Answer from the drawing. Dimensions are ordinates in mm from the lowest x, y and z of the part. A direction names the side the tool comes from. Coordinates: 2 decimals unless noted, no trailing zeros. Write each loop counter-clockwise with the first axis right and the second up, starting at its lowest first coordinate (ties: lowest second). Pieces come first, ordered by that corner, then holes.
(1) The part is cut by section B-B, the plane z = 1.5. State how many separate pieces and enclosed holes the cut face has, and give its area (3 significant figures).
(2) Given pin 1 (1.5 mm diameter, centred on x = 15.5, z = 4, fed in from -Y); pin 2 (3 mm diameter, centred on x = 13, z = 2, fed in from +Y); pin 3 (3 mm diameter, centred on x = 2, z = 2.5, fed in from +Y), each flat-ended and moving along its own axis, determine where each tip first touches the part or whether it passes through.
(3) The part is cut by section C-C, the plane x = 13.5. Determine the outline of the cut face in (y, z).
(4) The part is cut by section D-D, the plane x = 34. Determine the outline of the cut face in (y, z).
(5) Straight lines are drawn through the part: line 1 along X through (y, z) = (58.5, 4); line 2 along X through (y, z) = (39.5, 2.5) (1 decimal); line 3 along Y through (x, z) = (29.5, 5.5) (1 decimal). For each, find the intervals that lie inside material, in ascending order.
(6) The part is cut by section A-A, the plane x = 3. Determine the outline of the cut face in (y, z), and give its area (3 significant figures).
(7) Determine the mould class of the marked faces 1, 2 and 3 for opening direction Y: pulls with the +Y half, pulls with the -Y half, needs draft (parallel to the pull), parting line crosses it, or undercut.
(8) Which of the six approach directions +Z, -Z, +X, -X, +Y, -Y give full straight-line access (tool end or side, diameter ignored) to the marked faces 4 and 5?
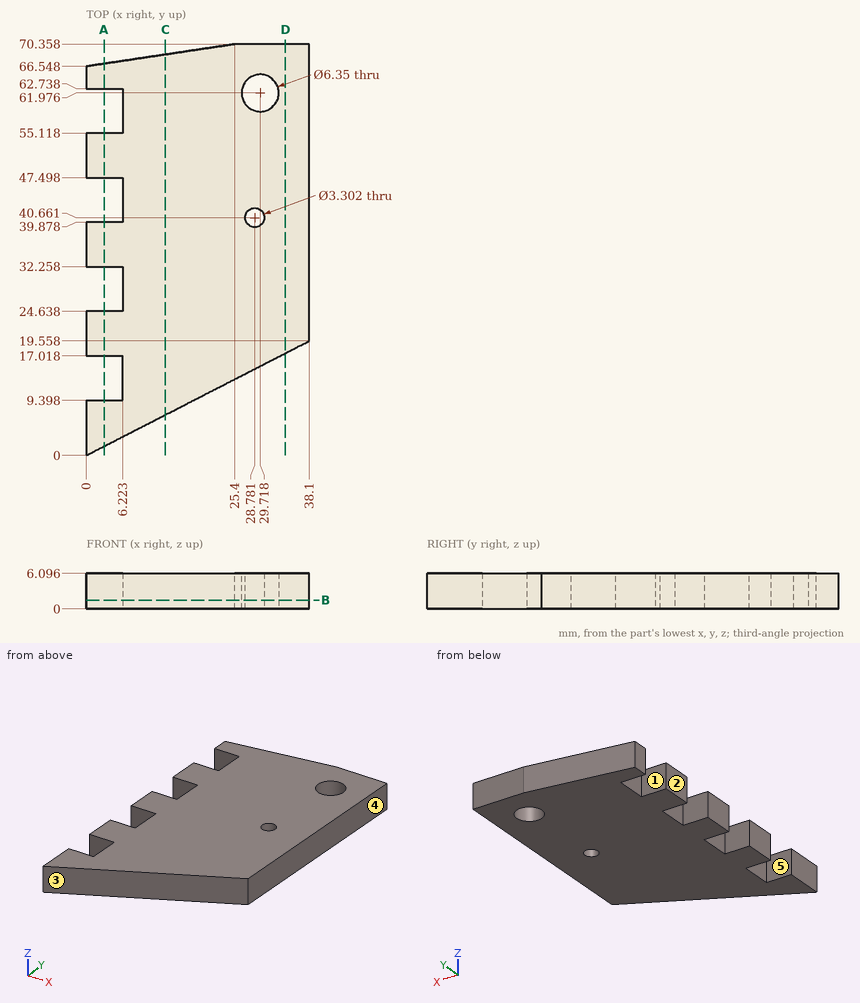
Computed:
1. separate pieces: 1
1. enclosed holes: 2
1. area: 2,030 mm2
2. pin 1: stops at y = 7.57
2. pin 2: stops at y = 68.72
2. pin 3: stops at y = 67.07
3. outline: (6.93, 0) - (68.57, 0) - (68.57, 6.1) - (6.93, 6.1) - close
4. outline: (17.45, 0) - (70.36, 0) - (70.36, 6.1) - (17.45, 6.1) - close
5. line 1: x = 6.22 to 38.1
5. line 2: x = 0 to 27.6, 30 to 38.1
5. line 3: y = 15.1 to 39.2, 42.1 to 58.8, 65.1 to 70.4
6. outline: (1.54, 0) - (9.4, 0) - (9.4, 6.1) - (1.54, 6.1) - close; (17.02, 0) - (24.64, 0) - (24.64, 6.1) - (17.02, 6.1) - close; (32.26, 0) - (39.88, 0) - (39.88, 6.1) - (32.26, 6.1) - close; (47.5, 0) - (55.12, 0) - (55.12, 6.1) - (47.5, 6.1) - close; (62.74, 0) - (67, 0) - (67, 6.1) - (62.74, 6.1) - close
6. area: 213 mm2
7. face 1: undercut
7. face 2: needs draft
7. face 3: pulls with the -Y half
8. face 4: +Z, -Z, +X, +Y, -Y
8. face 5: +Z, -Z, -X
